Autodesk Inventor part; units mm, degrees
ref_plane "YZ Plane" through (0, 0, 0) normal (1, 0, 0) x (0, 1, 0)
ref_plane "XZ Plane" through (0, 0, 0) normal (0, 1, 0) x (-1, 0, 0)
ref_plane "XY Plane" through (0, 0, 0) normal (0, 0, 1) x (1, 0, 0)
sketch "스케치1" plane through (0, 0, 0) normal (0, 0, 1) x (1, 0, 0)
  circle A0 centre (0, 0) radius 18
  circle A1 centre (0, 0) radius 16
  dimension "d0" = 36
  dimension "d1" = 32
extrude "돌출1" add sketch "스케치1" along normal mid plane 500
sketch "스케치2" plane through (0, 0, 250) normal (0, 0, 1) x (1, 0, 0)
  line L0 (-25, 18) -> (25, 18)
  line L1 (25, 18) -> (25, -18)
  line L2 (25, -18) -> (-25, -18)
  line L3 (-25, -18) -> (-25, 18)
  line L4 (-25, 18) -> (25, -18) construction
  line L5 (25, 18) -> (-25, -18) construction
  point P0 (0, 0)
  dimension "d4" = 50
extrude "돌출2" add sketch "스케치2" along normal blind 70
sketch "스케치3" plane through (0, 0, 320) normal (0, 0, 1) x (1, 0, 0)
  circle A0 centre (0, 0) radius 16
extrude "돌출3" cut sketch "스케치3" against normal blind 70
properties part number "motor_arm"
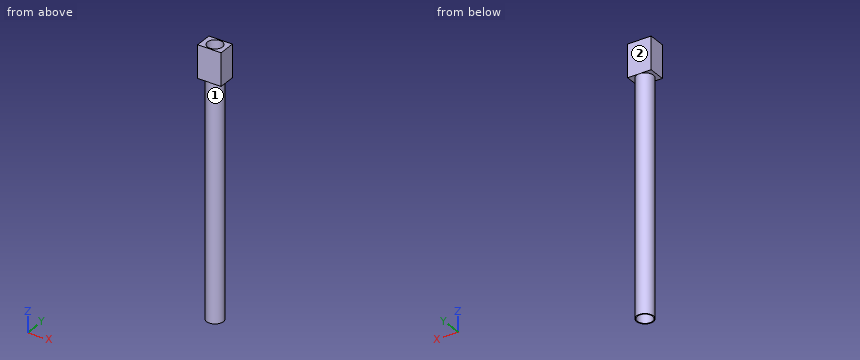
Build history of the part. All positions in model axes, mm. Face numbers are marked on the shaded views. A direction names the side the tool comes from. Give positions to 0.01 mm unless a question says otherwise; leave off trailing zeros. Order: outer loops, then holes, each group sorted by start corner. A loop starts at its lowest first (then second) coordinate and runs counter-clockwise, first axis right, second up. Notation, with made-up numbers: M 65.5,24 L 118.5,24 A7 ccw 118.5,29 Z; hole C 54.25,-28 d9. An arc over 180 degrees is marked long. Return JSON: item names as keys, results as strings.
Q1. Band-saw the part on A-A (z = 37.5). Give the cut face in (x, y), then the cut area to 3 significant figures.
Answer list:
{"outline": "C 0,0 d36; hole C 0,0 d32", "area": "214 mm^2"}
Q2. Band-saw the part on B-B (x = -8.5). Give the cut face in (y, z).
Answer list:
{"outline": "M -18,250 L -15.87,250 L -15.87,-250 L -13.56,-250 L -13.56,320 L -18,320 Z; M 13.56,-250 L 15.87,-250 L 15.87,250 L 18,250 L 18,320 L 13.56,320 Z"}
Q3. Wall check: probe 1 along Y at (x, z) = (0, 171); probe 2 along X at (y, z) = (13, 55); probe 3 along X at (y, z) = (9.5, -210.5). Give the ranges that are in metal, low to high. Write a range as from..to.
Answer list:
{"probe 1": "y = -18..-16, 16..18", "probe 2": "x = -12.45..-9.33, 9.33..12.45", "probe 3": "x = -15.29..-12.87, 12.87..15.29"}
Q4. Band-saw the part on C-C (y = -8). Give the cut face in (x, z).
Answer list:
{"outline": "M -25,250 L -16.12,250 L -16.12,-250 L -13.86,-250 L -13.86,320 L -25,320 Z; M 13.86,-250 L 16.12,-250 L 16.12,250 L 25,250 L 25,320 L 13.86,320 Z"}
Q5. Flat gauge pins, fed straight in: pin 1 (12 mm diameter, centred on x = 15.5, z = 63, fed in from +Y); pin 2 (5 mm diameter, centred on x = -19, y = -9.5, fed in from -Z); pin 3 (1.5 mm diameter, centred on x = 17, z = 50.5, fed in from -Y). Where does each tip first touch, or does it go through?
Answer list:
{"pin 1": "stops at y = 15.29", "pin 2": "stops at z = 250", "pin 3": "stops at y = -7.74"}
Q6. 3-axis set-ups, long thin cutter, end or side, ignore diameter. For the marked faces 1 and 2: which of +Z, -Z, +X, -X, +Y, -Y reach the whole face in a straight line?
Answer list:
{"face 1": "-Z", "face 2": "+Z, -Z, +X, -X, +Y"}
